from build123d import *

# Parameters (mm, degrees)
SKETCH1_R           = 5
BOSS_EXTRUDE1_DEPTH = 10
FILLET1_R           = 2.54
SCALE1_SCALE        = 0.66


with BuildPart() as part:
    # Sketch1 → Boss-Extrude1 (new body)
    with BuildSketch(Plane(origin=(0, 0, 0), x_dir=(1, 0, 0), z_dir=(0, 1, 0))):
        with BuildLine():
            Line((-3.580776184, -6.25), (34.060776184, -6.25))
            ThreePointArc((34.060776184, -6.25), (37.122638362, -6.730283618), (39.890388092, -8.125))
            ThreePointArc((39.890388092, -8.125), (55.72, 0), (39.890388092, 8.125))
            ThreePointArc((39.890388092, 8.125), (37.122638362, 6.730283618), (34.060776184, 6.25))
            Line((34.060776184, 6.25), (-3.580776184, 6.25))
            ThreePointArc((-3.580776184, 6.25), (-6.642638362, 6.730283618), (-9.410388092, 8.125))
            ThreePointArc((-9.410388092, 8.125), (-25.24, 0), (-9.410388092, -8.125))
            ThreePointArc((-9.410388092, -8.125), (-6.642638362, -6.730283618), (-3.580776184, -6.25))
        make_face()
        with Locations((-15.24, 0)):
            Circle(SKETCH1_R, mode=Mode.SUBTRACT)
        with Locations((45.72, 0)):
            Circle(SKETCH1_R, mode=Mode.SUBTRACT)
    extrude(amount=BOSS_EXTRUDE1_DEPTH)

    # Fillet1
    fillet1_edges = [part.edges().sort_by_distance(p)[0] for p in [
        (-6.642638362, 10, 6.730283618),
        (-25.24, 0, 0),
        (-6.642638362, 0, -6.730283618),
        (15.24, 10, 6.25),
        (37.122638362, 10, 6.730283618),
        (55.72, 10, 0),
        (37.122638362, 10, -6.730283618),
        (15.24, 10, -6.25),
        (-6.642638362, 10, -6.730283618),
        (-25.24, 10, 0),
        (15.24, 0, -6.25),
        (37.122638362, 0, -6.730283618),
        (55.72, 0, 0),
        (37.122638362, 0, 6.730283618),
        (15.24, 0, 6.25),
        (-6.642638362, 0, 6.730283618),
    ]]
    fillet(fillet1_edges, radius=FILLET1_R)


with BuildPart() as part_1:
    # Scale1: scaled about (15.24, 5, 0)
    add(part.part.scale(SCALE1_SCALE).moved(Location((5.1816, 1.7, 0))))


solid = part_1.part
Geometry: final body of the model. Coordinates: model frame, mm. A direction names the side the tool comes from. Coordinates: 2 decimals unless noted, no trailing zeros. Loops run counter-clockwise (first coordinate to the right, second up) from the corner with the lowest first, then second, coordinate; pieces in that order, holes last. Notation, with made-up numbers: (-18.5, 47.25) - (40.5, 47.25) arc R29 cw to (40.5, 79.25) - close; hole circle Ø11 at (-6, 71). An arc over 180 degrees is marked (long way). Put each result on its own line as item: value. Start each with the question number.
Q1. Cut plane A-A, the plane z = 0. Return loops of the section in (x, y).
Q2. Cut plane C-C, the plane x = 4. Return loops of the section in (y, z) (3 decimals), and give its area (3 significant figures).
Q3. Cut plane B-B, the plane y = 4.25. Return loops of the section in (x, z) (1 decimal).
Q4. Cut plane D-D, the plane y = 7.5. Return loops of the section in (x, z) (3 decimals), and give its area (3 significant figures).
Q5. Line query: line 1 (X direction, y = 5.5, z = 0); line 2 (X direction, y = 6, z = -0.25); line 3 (Z direction, x = 7, y = 4.25) (3 decimals). Output: solid intervals per line, ascending.
Q6. Pull-direction query (X, two-part tool) for faces 1 (the cylindrical face through (15.066, 7.796, -3.647)), 2 (the cylindrical face through (15.414, 2.204, 3.647)), 3 (the flat face through (15, 8.3, 0)); classes: released by +X, released by -X, zero draft, split by the parting line, or undercut.
Q7. Set-up query: faces 4 (the flat face through (15, 5, 4.125)), 5 (the cylindrical face through (15.066, 2.204, -3.647)), 6 (the flat face through (15, 5, -4.125)), 7 (the cylindrical face through (15.414, 7.796, 3.647)). Return all of +Z, -Z, +X, -X, +Y, -Y with unobstructed straight access to the full face (end or side cutting, diameter ignored); none if empty.
Q8. Pin query (flat end, axial travel): pin 1 Ø2.5 at (x, y) = (15, 5) entering from -Z (3 decimals); pin 2 Ø3.5 at (x, y) = (10, 4) entering from +Z (3 decimals); pin 3 Ø1.5 at (y, z) = (7.5, -5) entering from +X; pin 4 Ø5.5 at (x, z) = (-4.88, 0) entering from +Y. Return the tip coordinate at first contact, or that it passes through.
Filled sheet:
1. outline: (-11.48, 3.38) arc R1.68 ccw to (-9.8, 1.7) - (-8.18, 1.7) - (-8.18, 8.3) - (-9.8, 8.3) arc R1.68 ccw to (-11.48, 6.62) - close; (-1.58, 1.7) - (32.06, 1.7) - (32.06, 8.3) - (-1.58, 8.3) - close; (38.66, 1.7) - (40.28, 1.7) arc R1.68 ccw to (41.96, 3.38) - (41.96, 6.62) arc R1.68 ccw to (40.28, 8.3) - (38.66, 8.3) - close
2. outline: (1.7, -2.449) arc R1.676 ccw to (3.376, -4.125) - (6.624, -4.125) arc R1.676 ccw to (8.3, -2.449) - (8.3, 2.449) arc R1.676 ccw to (6.624, 4.125) - (3.376, 4.125) arc R1.676 ccw to (1.7, 2.449) - close
2. area: 52.0 mm²
3. outline: (-1, -5.4) arc R6.6 cw to (2.8, -4.1) - (27.7, -4.1) arc R6.6 cw to (31.5, -5.4) arc R6.6 ccw (long way) to (31.5, 5.4) arc R6.6 cw to (27.7, 4.1) - (2.8, 4.1) arc R6.6 cw to (-1, 5.4) arc R6.6 ccw (long way) to start; hole circle Ø6.6 at (-4.9, 0); hole circle Ø6.6 at (35.4, 0)
4. outline: (-1.173, -5.162) arc R6.847 cw to (2.818, -3.878) - (27.662, -3.878) arc R6.847 cw to (31.653, -5.162) arc R6.353 ccw (long way) to (31.653, 5.162) arc R6.847 cw to (27.662, 3.878) - (2.818, 3.878) arc R6.847 cw to (-1.173, 5.162) arc R6.353 ccw (long way) to start; hole circle Ø6.6 at (-4.877, 0); hole circle Ø6.6 at (35.357, 0)
4. area: 408 mm²
5. line 1: -11.48 to -8.18, -1.58 to 32.06, 38.66 to 41.96
5. line 2: -11.47 to -8.17, -1.59 to 32.07, 38.65 to 41.95
5. line 3: -4.125 to 4.125
6. face 1: undercut
6. face 2: undercut
6. face 3: zero draft
7. face 4: +Z, +Y, -Y
7. face 5: -Z, -Y
7. face 6: -Z, +Y, -Y
7. face 7: +Z, +Y
8. pin 1: z = -4.125
8. pin 2: z = 4.125
8. pin 3: x = 40.22
8. pin 4: through
